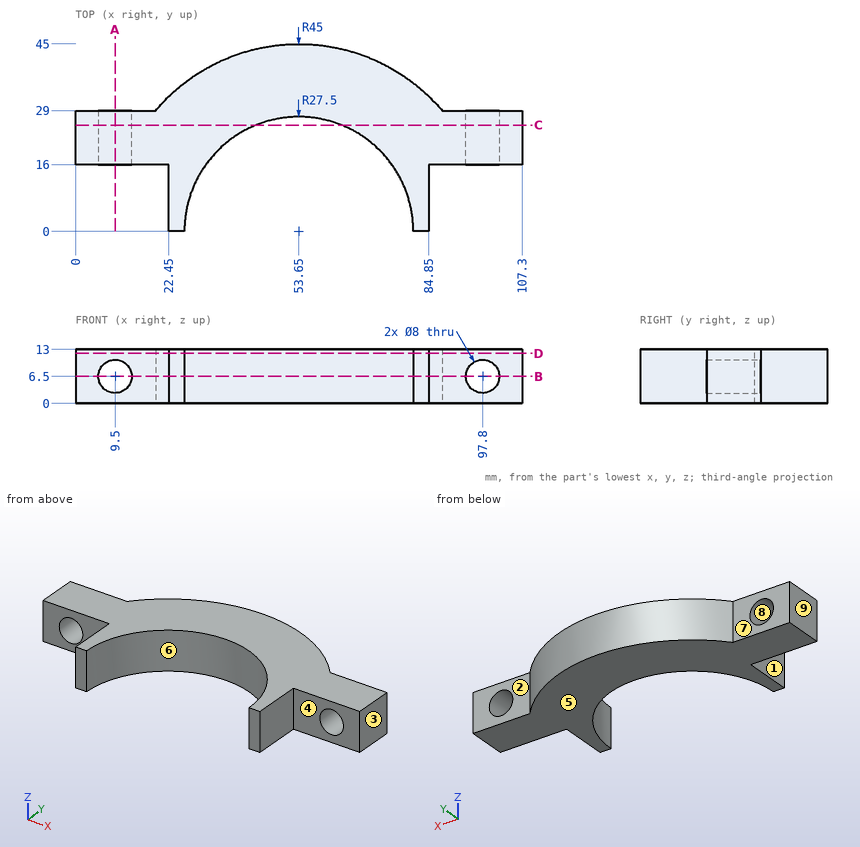
Here's the drawing with two shaded views (mm, measured from the low corner). I have some questions. A direction names the side the tool comes from. Round coordinates to 2 decimals unless told otherwise and drop trailing zeros. Order: outer loops, then holes, each group sorted by start corner. A loop starts at its lowest first (then second) coordinate and runs counter-clockwise, first axis right, second up. Notation, with made-up numbers: (11.25, 46.5) -> (69.25, 46.5) arc R15 cw to (69.25, 74.5) -> close; hole circle Ø6 at (-38.5, 27). An arc over 180 degrees is marked (long way). Use a Markdown table: item, result. Add a question column.
(1) Suppose I cut it at B-B, the plane z = 6.5. Please give me the cut outline in (x, y), and give its area (3 significant figures).
(2) I need wall thicknesses on line 1 along Z through (x, y) = (9.5, 23); line 2 along X through (y, z) = (10.5, 12); line 3 along X through (y, z) = (4, 12.25). Which ranges of each line are inside material? Lowest first, please.
(3) Suppose I cut it at C-C, the plane y = 25.5. Please give me the cut outline in (x, z), and give its area (3 significant figures).
(4) For pin 1 Ø6.5 at (y, z) = (6.5, 4) entering from +X; pin 2 Ø6.5 at (x, z) = (13.5, 6) entering from -Y; pin 3 Ø4 at (y, z) = (10.5, 8) entering from -X, each with a flat end and sliding along its axis, tell me the tip position at first contact or that it passes through.
(5) Suppose I cut it at A-A, the plane x = 9.5. Please give me the cut outline in (y, z), and give its area (3 significant figures).
(6) For the marked faces 1, 2, 3, 4 and 5, which set-ups out of +Z, -Z, +X, -X, +Y, -Y let a thin tool reach every point of the face, with its end or its side?
(7) Suppose I cut it at D-D, the plane z = 12. Please give me the cut outline in (x, y).
(8) If we mould it in two halves opening along X, with no side actions, what happens to the marked faces 6, 7, 8 and 9? For each: released by +X, released by -X, zero draft, split by the parting line, or undercut.
Verdict:
| question | item | result |
|---|---|---|
| 1 | outline | (0, 16) -> (5.5, 16) -> (5.5, 29) -> (0, 29) -> close; (13.5, 16) -> (22.45, 16) -> (22.45, 0) -> (26.15, 0) arc R27.5 cw to (81.15, 0) -> (84.85, 0) -> (84.85, 16) -> (93.8, 16) -> (93.8, 29) -> (88.06, 29) arc R45 ccw to (19.24, 29) -> (13.5, 29) -> close; (101.8, 16) -> (107.3, 16) -> (107.3, 29) -> (101.8, 29) -> close |
| 1 | area | 1,760 mm2 |
| 2 | line 1 | 0 to 2.5, 10.5 to 13 |
| 2 | line 2 | 22.45 to 28.23, 79.07 to 84.85 |
| 2 | line 3 | 22.45 to 26.44, 80.86 to 84.85 |
| 3 | outline | (0, 0) -> (43.35, 0) -> (43.35, 13) -> (0, 13) -> close; (63.95, 0) -> (107.3, 0) -> (107.3, 13) -> (63.95, 13) -> close; hole circle Ø8 at (9.5, 6.5); hole circle Ø8 at (97.8, 6.5) |
| 3 | area | 1,030 mm2 |
| 4 | pin 1 | x = 84.85 |
| 4 | pin 2 | y = 16 |
| 4 | pin 3 | x = 22.45 |
| 5 | outline | (16, 0) -> (29, 0) -> (29, 2.5) -> (16, 2.5) -> close; (16, 10.5) -> (29, 10.5) -> (29, 13) -> (16, 13) -> close |
| 5 | area | 65.0 mm2 |
| 6 | face 1 | +Z, -Z, -X, -Y |
| 6 | face 2 | +Z, -Z, +X, +Y |
| 6 | face 3 | +Z, -Z, +X, +Y, -Y |
| 6 | face 4 | +Z, -Z, +X, -Y |
| 6 | face 5 | -Z, +X, -X, +Y, -Y |
| 7 | outline | (0, 16) -> (22.45, 16) -> (22.45, 0) -> (26.15, 0) arc R27.5 cw to (81.15, 0) -> (84.85, 0) -> (84.85, 16) -> (107.3, 16) -> (107.3, 29) -> (88.06, 29) arc R45 ccw to (19.24, 29) -> (0, 29) -> close |
| 8 | face 6 | undercut |
| 8 | face 7 | zero draft |
| 8 | face 8 | undercut |
| 8 | face 9 | released by -X |
